The figure shows three views and two pictorial views of one solid part (mm, origin at its lowest corner). Answer the questions. A direction names the side the tool comes from. Give positions to 0.01 mm unless a question says otherwise; leave off trailing zeros. Loops run counter-clockwise (first coordinate to the right, second up) from the corner with the lowest first, then second, coordinate; pieces in that order, holes last. Notation, with made-up numbers: (-23.75, 29) -> (29.25, 29) arc R34 ccw to (29.25, 67) -> close; hole circle Ø3 at (71.25, 65.5). An arc over 180 degrees is marked (long way). Answer as CSV lines item,"result". Start each with the question number.
1. A tool of negligible diameter and unlimited length cuts with its end or side. For the marked faces 1 and 2, from which of +Z, -Z, +X, -X, +Y, -Y can it reach the whole face along a straight path? Write none if from no direction.
2. Find section C-C, the plane y = 13.5. Give the vertices of the cut face in (x, z), and give its area (3 significant figures).
3. Flat-ended cylindrical pins translate along their axes: pin 1 Ø12 at (y, z) = (24, 14) entering from +X; pin 2 Ø1.5 at (y, z) = (26.5, 20.5) entering from +X; pin 3 Ø10 at (x, z) = (32, 26) entering from +Y; pin 4 Ø2.5 at (x, z) = (5.5, 5.5) entering from -Y. Find the tip coordinate at first contact, or state that the pin passes through.
4. Find the intervals of material crossed by line 1 along Z through (x, y) = (5, 13); line 2 along X through (y, z) = (9.75, 36.5); line 3 along Y through (x, z) = (11, 8), in increasing order.
5. Find section D-D, the plane x = 21. Give the vertices of the cut face in (y, z), and give its area (3 significant figures).
6. Find section A-A, the plane z = 36.5. Give the vertices of the cut face in (x, y).
7. Find section B-B, the plane x = 5.5. Give the vertices of the cut face in (y, z), and give its area (3 significant figures).
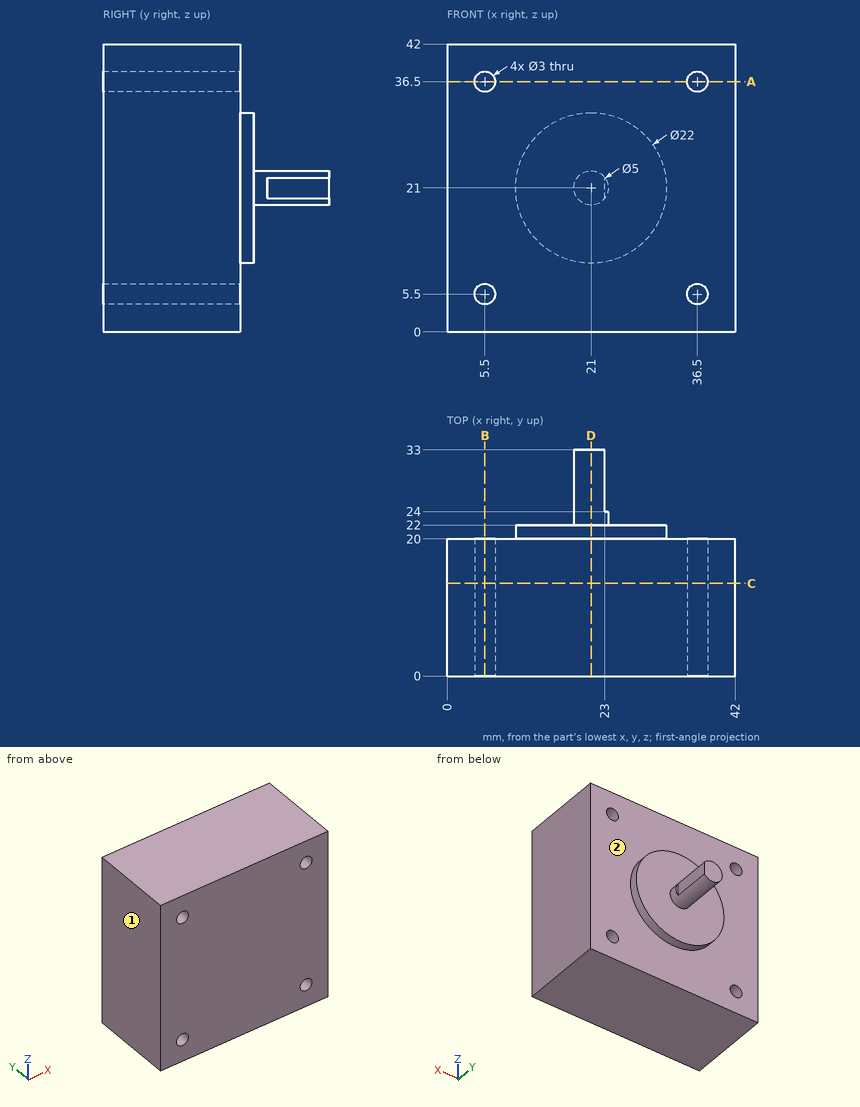
Resolved:
1,face 1,"+Z, -Z, -X, +Y, -Y"
1,face 2,"+Y"
2,outline,"(0, 0) -> (42, 0) -> (42, 42) -> (0, 42) -> close; hole circle Ø3 at (5.5, 5.5); hole circle Ø3 at (5.5, 36.5); hole circle Ø3 at (36.5, 5.5); hole circle Ø3 at (36.5, 36.5)"
2,area,"1,740 mm^2"
3,pin 1,"stops at x = 42"
3,pin 2,"stops at x = 23"
3,pin 3,"stops at y = 22"
3,pin 4,"passes through"
4,line 1,"z = 0 to 4.09, 6.91 to 35.09, 37.91 to 42"
4,line 2,"x = 0 to 4, 7 to 35, 38 to 42"
4,line 3,"y = 0 to 20"
5,outline,"(0, 0) -> (20, 0) -> (20, 10) -> (22, 10) -> (22, 18.5) -> (33, 18.5) -> (33, 23.5) -> (22, 23.5) -> (22, 32) -> (20, 32) -> (20, 42) -> (0, 42) -> close"
5,area,"939 mm^2"
6,outline,"(0, 0) -> (4, 0) -> (4, 20) -> (0, 20) -> close; (7, 0) -> (35, 0) -> (35, 20) -> (7, 20) -> close; (38, 0) -> (42, 0) -> (42, 20) -> (38, 20) -> close"
7,outline,"(0, 0) -> (20, 0) -> (20, 4) -> (0, 4) -> close; (0, 7) -> (20, 7) -> (20, 35) -> (0, 35) -> close; (0, 38) -> (20, 38) -> (20, 42) -> (0, 42) -> close"
7,area,"720 mm^2"
